```python
from build123d import *

# Parameters (mm, degrees)
BOSS_EXTRU_1_DEPTH           = 13
ENL_V_MAT_EXTRU_1_DEPTH      = 91.210864091
ENL_V_MAT_EXTRU_1_DEPTH_BACK = 91.210864091
ESQUISSE2_R                  = 4


with BuildPart() as part:
    # Esquisse1 → Boss.-Extru.1 (new body)
    with BuildSketch(Plane.XY):
        with BuildLine():
            Line((0, 15), (80, 8))
            ThreePointArc((80, 8), (88, 0), (80, -8))
            Line((80, -8), (0, -15))
            ThreePointArc((0, -15), (-15, 0), (0, 15))
        make_face()
    extrude(amount=BOSS_EXTRU_1_DEPTH)

    # Esquisse2 → Enlèv. mat.-Extru.1 (cut, two sides: drawn at the far end of the back side and taken through both)
    with BuildSketch(Plane.XY.offset(13).offset(-ENL_V_MAT_EXTRU_1_DEPTH_BACK)):
        with Locations((-3, 3)):
            Circle(ESQUISSE2_R)
    extrude(amount=ENL_V_MAT_EXTRU_1_DEPTH + ENL_V_MAT_EXTRU_1_DEPTH_BACK, mode=Mode.SUBTRACT)


solid = part.part
```
The listing builds one solid part. Answer for the finished solid, in the listing's coordinates (mm). Give positions to 0.01 mm unless a question says otherwise; leave off trailing zeros. Order: outer loops, then holes, each group sorted by start corner. A loop starts at its lowest first (then second) coordinate and runs counter-clockwise, first axis right, second up. Notation, with made-up numbers: (33, 45) -> (59, 45) arc R22 ccw to (59, 79) -> close; hole circle Ø9 at (26, -24). An arc over 180 degrees is marked (long way). Answer as a JSON object with one key per item and string values. Group by question number.
Item 1: The part is cut by section A-A on z = 7.75. Write down the section's boundary in (x, y).
Item 2: Determine the mould class of faces 1 (the flat face through (37, 0, 13)), 2 (the flat face through (39.44, 11.55, 6.41)), 3 (the cylindrical face through (-15, 0, 6)), 4 (the cylindrical face through (-3.867, -0.905, 6.409)) for opening direction X: pulls with the +X half, pulls with the -X half, needs draft (parallel to the pull), parting line crosses it, or undercut.
Item 3: The part is cut by section B-B on y = 0. Write down the section's boundary in (x, z).
Item 4: Flat-ended cylindrical pins translate along their axes: pin 1 (1.5 mm diameter, centred on x = 69.5, z = 3, fed in from +Y); pin 2 (2 mm diameter, centred on y = 7.5, z = 8, fed in from -X); pin 3 (4 mm diameter, centred on y = 8.5, z = 10, fed in from +X); pin 4 (7 mm diameter, centred on x = -3, y = 3, fed in from -Z). Find the tip coordinate at first contact, or state that the pin passes through.
Item 5: The part is cut by section C-C on x = -3. Write down the section's boundary in (y, z), and give its area (3 significant figures).
Item 6: The part is cut by section D-D on x = 32. Write down the section's boundary in (y, z).
Item 7: Consider L1, parallel to Y at x = -3, z = 9.5; L2, parallel to X at y = 3, z = 3; L3, parallel to Y at x = 80.5, z = 7.75. Determine where each line is inside the solid, lowest interval first. Write a range as from..to.
Result set:
{
 "1": {"outline": "(0, -15) -> (80, -8) arc R8 ccw to (80, 8) -> (0, 15) arc R15 ccw to start; hole circle Ø8 at (-3, 3)"},
 "2": {"face 1": "needs draft", "face 2": "pulls with the +X half", "face 3": "pulls with the -X half", "face 4": "undercut"},
 "3": {"outline": "(-15, 0) -> (-5.65, 0) -> (-5.65, 13) -> (-15, 13) -> close; (-0.35, 0) -> (88, 0) -> (88, 13) -> (-0.35, 13) -> close"},
 "4": {"pin 1": "y = 8.98", "pin 2": "x = -13.52", "pin 3": "x = 84.66", "pin 4": "through"},
 "5": {"outline": "(-14.7, 0) -> (-1, 0) -> (-1, 13) -> (-14.7, 13) -> close; (7, 0) -> (14.7, 0) -> (14.7, 13) -> (7, 13) -> close", "area": "278 mm²"},
 "6": {"outline": "(-12.2, 0) -> (12.2, 0) -> (12.2, 13) -> (-12.2, 13) -> close"},
 "7": {"L1": "-14.7..-1, 7..14.7", "L2": "-14.7..-7, 1..87.42", "L3": "-7.98..7.98"}
}
